Design review of the part built by this model. Coordinates are the model's own, in mm. Coordinates: 2 decimals unless noted, no trailing zeros. Answer in a Markdown table with one row per item. Add a question column.
(1) The part is to be moulded in two halves that separate along Y. For faces 1 (the face through (-7.709, -34.714, 62.611)), 2 (the face through (0, 0, 127)), 3 (the face through (0, 0, 152.4)), 4 (the face through (-6.607, 29.755, 62.611)), say which applies: released by +Y, released by -Y, zero draft, split by the parting line, or undercut.
(2) Clearance check with flat-ended pins moving along their axes: pin 1 (2 mm diameter, centred on x = -13, y = -21, fed in from -Z); pin 2 (3 mm diameter, centred on x = 1.5, z = 108.5, fed in from +Y); pin 3 (5 mm diameter, centred on y = -12, z = 32.5, fed in from +X). State where each tip first meets the part, or that it passes through.
(3) To check wall thickness, follow L1, parallel to Y at x = 0, z = 44; L2, parallel to Y at x = -20.5, z = 27.5; L3, parallel to X at y = -4, z = 39. State the ranges of each line that lie inside material, in increasing order. Write a range as [from, to].
from build123d import *

# Parameters (mm, degrees)
F0_R     = 35.56
F1_DEPTH = 127
F2_DEPTH = 25.4
F3_R     = 25.4
F4_R     = 30.48
F5_DEPTH = 127


with BuildPart() as f1:
    # F0 (on Top) → F1 (new body)
    with BuildSketch(Plane.XY):
        Circle(F0_R)
    extrude(amount=F1_DEPTH)

    # F2 (add): a face of the model
    f2_faces = [f1.faces().sort_by_distance(p)[0] for p in [
        (0, 0, 127),
    ]]
    extrude(f2_faces, amount=F2_DEPTH)

    # F3
    f3_edges = [f1.edges().sort_by_distance(p)[0] for p in [
        (-35.56, 0, 152.4),
    ]]
    fillet(f3_edges, radius=F3_R)

    # F4 (on face) → F5 (cut)
    with BuildSketch(Plane(origin=(0, 0, 0), x_dir=(1, 0, 0), z_dir=(0, 0, -1))):
        Circle(F4_R)
    extrude(amount=-F5_DEPTH, mode=Mode.SUBTRACT)


solid = f1.part
Responses:
| question | item | result |
|---|---|---|
| 1 | face 1 | split by the parting line |
| 1 | face 2 | undercut |
| 1 | face 3 | zero draft |
| 1 | face 4 | undercut |
| 2 | pin 1 | stops at z = 127 |
| 2 | pin 2 | stops at y = 35.56 |
| 2 | pin 3 | stops at x = 34.27 |
| 3 | L1 | y = [-35.56, -30.48], [30.48, 35.56] |
| 3 | L2 | y = [-29.06, -22.56], [22.56, 29.06] |
| 3 | L3 | x = [-35.33, -30.22], [30.22, 35.33] |
